Autodesk Inventor part; units mm, degrees
ref_plane "Startebene" through (0, 0, 0) normal (0, 0, 1) x (1, 0, 0)
ref_plane "Endebene" through (0, 0, 50) normal (0, 0, 1) x (1, 0, 0)
ref_plane "YZ Plane" through (0, 0, 0) normal (1, 0, 0) x (0, 1, 0)
ref_plane "Startebene" through (0, 0, 0) normal (0, 0, 1) x (1, 0, 0)
ref_plane "Endebene" through (0, 0, 50) normal (0, 0, 1) x (1, 0, 0)
sketch "Skizze" plane through (0, 0, 0) normal (0, 0, 1) x (1, 0, 0)
  line L0 (0, 0) -> (0, 100)
  line L1 (0, 100) -> (80, 100)
  line L2 (80, 100) -> (80, 89)
  line L3 (80, 89) -> (19, 89)
  line L4 (6, 76) -> (6, 0)
  line L5 (6, 0) -> (0, 0) construction
  line L6 (25.6, 100) -> (25.6, 89) construction
  line L7 (80, 89) -> (80, 89) construction
  line L8 (80, 89) -> (25.6, 89) construction
  line L9 (0, 12) -> (0, -30) construction
  line L10 (-1.5, 0) -> (19.5, 0) construction
  line L11 (0, 0) -> (0, -100)
  line L12 (0, -100) -> (80, -100)
  line L13 (80, -100) -> (80, -89)
  line L14 (80, -89) -> (19, -89)
  line L15 (6, -76) -> (6, 0)
  arc A0 (6, -76) -> (19, -89) centre (19, -76) ccw
  arc A1 (19, 89) -> (6, 76) centre (19, 76) ccw
  line L16 (0, 56) -> (0, -56) construction
  line L17 (-11.8, 0) -> (60.3, 0) construction
  point P0 (6, 89)
  point P1 (6, -89)
  point P2 (25.6, -100)
  point P3 (25.6, -89)
  dimension "d0" = 6
  dimension "d1" = 100
  dimension "d2" = 80
  dimension "d3" = 11
  dimension "d5" = 0
  dimension "d23" = 13
  dimension "d24" = 0
  dimension "d29" = 25.6
extrude "Körper" add sketch "Skizze" along normal up to surface (50 mm away) from surface at 0
sketch "Sketch3" plane through (0, 0, 0) normal (0, 0, 1) x (1, 0, 0)
  line L0 (0, 0) -> (10, 0)
ref_plane "Work Plane3" through (0, 0, 0) normal (0, -1, 0) x (1, 0, 0)
sketch "Sketch4" plane through (0, 0, 0) normal (0, -1, 0) x (1, 0, 0)
  line L0 (-2, 0) -> (12, 0)
  line L1 (-2, 50) -> (12, 50)
  dimension "d28" = 50
equation "\"d0\" = G_T"
equation "\"d1\" = 0.5 * G_H"
equation "\"d2\" = G_W"
equation "\"d3\" = G_T1"
equation "\"d23\" = G_IR"
equation "\"d29\" = G_C"
equation "\"d6\" = G_L"
equation "\"G_W\" = 80"
equation "\"G_T\" = 6"
equation "\"G_T1\" = 11"
equation "\"G_NG\" = 0"
equation "\"G_IR\" = 13"
equation "\"G_C\" = 25.6"
equation "\"G_L\" = d28"
equation "\"ex\" = 0"
equation "\"G_OFFSET_START\" = 0"
equation "\"G_OFFSET_END\" = 0"
properties part number "DIN 1026-2 - UPE 200 - 50" material "Stahl, weich"
Source: CAD feature listing. Evaluate the final solid. Frame: model axes, mm. A direction names the side the tool comes from. Give positions to 0.01 mm unless a question says otherwise; leave off trailing zeros. Order: outer loops, then holes, each group sorted by start corner. A loop starts at its lowest first (then second) coordinate and runs counter-clockwise, first axis right, second up. Notation, with made-up numbers: (-27, 32.25) -> (-2, 32.25) arc R23 cw to (-2, 57.25) -> close; hole circle Ø9 at (63, 28). An arc over 180 degrees is marked (long way). Write item = value, one per line.
Item 1: Set-up query: faces 5 (the face through (50, -89, 25)), 6 (the face through (80, 95, 25)). Return all of +Z, -Z, +X, -X, +Y, -Y with unobstructed straight access to the full face (end or side cutting, diameter ignored); none if empty.
Check result:
face_5 = +Z, -Z, +X
face_6 = +Z, -Z, +X, +Y, -Y
Item 2: Section query D-D (y = 25). Output: boundary loops of the cut face in (x, z), then the cut area to 3 significant figures.
Check result:
outline = (0, 0) -> (6, 0) -> (6, 50) -> (0, 50) -> close
area = 300 mm²
Item 3: Section query C-C (x = 14). Output: boundary loops of the cut face in (y, z), then the cut area to 3 significant figures.
Check result:
outline = (-100, 0) -> (-88, 0) -> (-88, 50) -> (-100, 50) -> close; (88, 0) -> (100, 0) -> (100, 50) -> (88, 50) -> close
area = 1,200 mm²
Item 4: Mould query, pull axis Y, two halves, no side actions, for faces 1 (the face through (39, 100, 25)), 2 (the face through (80, -95, 25)), 3 (the face through (50, 89, 25)), 4 (the face through (9.909, -85.293, 24.65)). Classes: +Y half, -Y half, draft (parallel to the pull), parting line (faces both ways), or undercut.
Check result:
face_1 = +Y half
face_2 = draft
face_3 = undercut
face_4 = undercut
Item 5: Section query A-A (x = 50). Output: boundary loops of the cut face in (y, z).
Check result:
outline = (-100, 0) -> (-89, 0) -> (-89, 50) -> (-100, 50) -> close; (89, 0) -> (100, 0) -> (100, 50) -> (89, 50) -> close
Item 6: Section query B-B (z = 36). Output: boundary loops of the cut face in (x, y), then the cut area to 3 significant figures.
Check result:
outline = (0, -100) -> (80, -100) -> (80, -89) -> (19, -89) arc R13 cw to (6, -76) -> (6, 76) arc R13 cw to (19, 89) -> (80, 89) -> (80, 100) -> (0, 100) -> close
area = 2,900 mm²
Item 7: Contact query for flat-ended pins moving along their axis: pin 1 (1 mm diameter, centred on y = -34.5, z = 43, fed in from +X); pin 2 (4 mm diameter, centred on y = 31, z = 9, fed in from -X). Output: stop coordinate, or through.
Check result:
pin_1 = 6
pin_2 = 0
Item 8: Ray query, probe 1 along Y at (x, z) = (32, 24.5); probe 2 along X at (y, z) = (-40.5, 30); probe 3 along Y at (x, z) = (11.5, 41). Return the intervals inside material, ascending.
Check result:
probe_1 = -100 to -89, 89 to 100
probe_2 = 0 to 6
probe_3 = -100 to -86.62, 86.62 to 100
